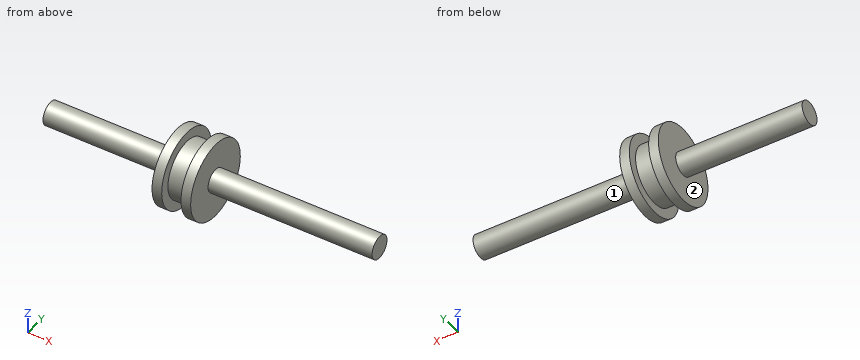
from build123d import *

# Parameters (mm, degrees)
SKETCH1_R           = 6
BOSS_EXTRUDE1_DEPTH = 65.5
SKETCH2_R           = 20
BOSS_EXTRUDE2_DEPTH = 5
SKETCH3_R           = 15
BOSS_EXTRUDE3_DEPTH = 10
SKETCH4_R           = 20
BOSS_EXTRUDE4_DEPTH = 5
SKETCH5_R           = 6
BOSS_EXTRUDE5_DEPTH = 85


with BuildPart() as part:
    # Sketch1 → Boss-Extrude1 (new body)
    with BuildSketch(Plane(origin=(0, 0, 0), x_dir=(0, 0, -1), z_dir=(1, 0, 0))):
        Circle(SKETCH1_R)
    extrude(amount=BOSS_EXTRUDE1_DEPTH)

    # Sketch2 → Boss-Extrude2 (add)
    with BuildSketch(Plane(origin=(65.5, 0, 0), x_dir=(0, 0, -1), z_dir=(1, 0, 0))):
        Circle(SKETCH2_R)
    extrude(amount=BOSS_EXTRUDE2_DEPTH)

    # Sketch3 → Boss-Extrude3 (add)
    with BuildSketch(Plane(origin=(70.5, 0, 0), x_dir=(0, 0, -1), z_dir=(1, 0, 0))):
        Circle(SKETCH3_R)
    extrude(amount=BOSS_EXTRUDE3_DEPTH)

    # Sketch4 → Boss-Extrude4 (add)
    with BuildSketch(Plane(origin=(80.5, 0, 0), x_dir=(0, 0, -1), z_dir=(1, 0, 0))):
        Circle(SKETCH4_R)
    extrude(amount=BOSS_EXTRUDE4_DEPTH)

    # Sketch5 → Boss-Extrude5 (add)
    with BuildSketch(Plane(origin=(85.5, 0, 0), x_dir=(0, 0, -1), z_dir=(1, 0, 0))):
        Circle(SKETCH5_R)
    extrude(amount=BOSS_EXTRUDE5_DEPTH)


solid = part.part
Geometry check sheet. Reference: the model listing, model coordinates, mm. Face numbers are marked on the shaded views. A direction names the side the tool comes from. Give positions to 0.01 mm unless a question says otherwise; leave off trailing zeros. Loops run counter-clockwise (first coordinate to the right, second up) from the corner with the lowest first, then second, coordinate; pieces in that order, holes last. Notation, with made-up numbers: (36.25, 83) -> (93.25, 83) arc R5 cw to (93.25, 88) -> close; hole circle Ø2 at (-19.5, 76.5). An arc over 180 degrees is marked (long way). Answer in a Markdown table with one row per item. Add a question column.
1) Cross-section at D-D on z = 9. Record the boundary of the cut face in (x, y).
2) Set-up check for the marked faces 1 and 2: record each of +Z, -Z, +X, -X, +Y, -Y from which the full face is reachable in a straight line by a thin tool's end or side.
3) Material ranges on probe 1 along X at (y, z) = (-0.5, -15.5); probe 2 along Y at (x, z) = (48.5, -0.5), recorded low to high. Write a range as from..to.
4) Cross-section at C-C on x = 137.5. Record the boundary of the cut face in (y, z).
5) Gauge pin test, flat ends, axial feed: P1, Ø8, axis at x = 150.5, z = 6, coming from the +Y side; P2, Ø12, axis at y = 7.5, z = -3, coming from the -X side; P3, Ø1, axis at x = 145, y = 5.5, coming from the -Z side; P4, Ø1, axis at x = 68, y = 7.5, coming from the -Z side (3 decimals). Record the tip position at first contact, or that the pin passes through.
6) Cross-section at B-B on z = 0. Record the boundary of the cut face in (x, y), and give its area (3 significant figures).
7) Cross-section at A-A on y = -12. Record the boundary of the cut face in (x, z).
Outcome:
| question | item | result |
|---|---|---|
| 1 | outline | (65.5, -17.86) -> (70.5, -17.86) -> (70.5, -12) -> (80.5, -12) -> (80.5, -17.86) -> (85.5, -17.86) -> (85.5, 17.86) -> (80.5, 17.86) -> (80.5, 12) -> (70.5, 12) -> (70.5, 17.86) -> (65.5, 17.86) -> close |
| 2 | face 1 | +X |
| 2 | face 2 | -X |
| 3 | probe 1 | x = 65.5..70.5, 80.5..85.5 |
| 3 | probe 2 | y = -5.98..5.98 |
| 4 | outline | circle Ø12 at (0, 0) |
| 5 | P1 | stops at y = 5.66 |
| 5 | P2 | stops at x = 0 |
| 5 | P3 | stops at z = -3.32 |
| 5 | P4 | stops at z = -18.735 |
| 6 | outline | (0, -6) -> (65.5, -6) -> (65.5, -20) -> (70.5, -20) -> (70.5, -15) -> (80.5, -15) -> (80.5, -20) -> (85.5, -20) -> (85.5, -6) -> (170.5, -6) -> (170.5, 6) -> (85.5, 6) -> (85.5, 20) -> (80.5, 20) -> (80.5, 15) -> (70.5, 15) -> (70.5, 20) -> (65.5, 20) -> (65.5, 6) -> (0, 6) -> close |
| 6 | area | 2,510 mm^2 |
| 7 | outline | (65.5, -16) -> (70.5, -16) -> (70.5, -9) -> (80.5, -9) -> (80.5, -16) -> (85.5, -16) -> (85.5, 16) -> (80.5, 16) -> (80.5, 9) -> (70.5, 9) -> (70.5, 16) -> (65.5, 16) -> close |
